Work out the finished part from the listing and answer in its coordinate system (mm). Face numbers are marked on the shaded views. A direction names the side the tool comes from. Coordinates: 2 decimals unless noted, no trailing zeros. Write each loop counter-clockwise with the first axis right and the second up, starting at its lowest first coordinate (ties: lowest second). Pieces come first, ordered by that corner, then holes. Notation, with made-up numbers: (-23, 6.25) - (29, 6.25) arc R20 ccw to (29, 22.25) - close; hole circle Ø9 at (21.5, -31.5). An arc over 180 degrees is marked (long way). One line per item, written item: value.
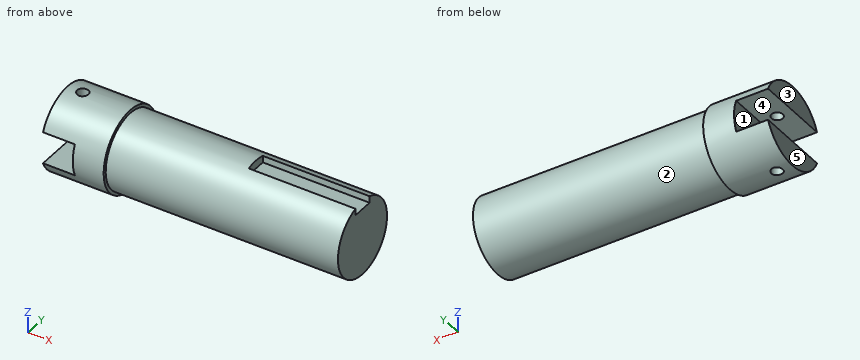
```python
from build123d import *

# Parameters (mm, degrees)
SKETCH1_R               = 30
BOSS_EXTRUDE1_DEPTH     = 185
SKETCH2_R               = 32.5
BOSS_EXTRUDE2_DEPTH     = 50
SKETCH3_W               = 17.227034698
SKETCH3_H               = 11
CUT_EXTRUDE1_DEPTH      = 85
SKETCH6_W               = 97.129715822
SKETCH6_H               = 25.4
CUT_EXTRUDE2_DEPTH      = 25.4
CUT_EXTRUDE3_DEPTH      = 66.4
CUT_EXTRUDE3_DEPTH_BACK = 25.4
SKETCH7_R               = 4.5


with BuildPart() as part:
    # Sketch1 → Boss-Extrude1 (new body)
    with BuildSketch(Plane.YZ):
        with Locations(Location((0, 0, 0), (0, 0, 270))):
            Circle(SKETCH1_R)
    extrude(amount=BOSS_EXTRUDE1_DEPTH)

    # Sketch2 → Boss-Extrude2 (add)
    with BuildSketch(Plane.ZY):
        Circle(SKETCH2_R)
    extrude(amount=BOSS_EXTRUDE2_DEPTH)

    # Sketch3 → Cut-Extrude1 (cut)
    with BuildSketch(Plane.YZ.offset(185)):
        with Locations((0, 28.9)):
            Rectangle(SKETCH3_W, SKETCH3_H)
    extrude(amount=-CUT_EXTRUDE1_DEPTH, mode=Mode.SUBTRACT)

    # Sketch6 → Cut-Extrude2 (cut)
    with BuildSketch(Plane(origin=(-50, 0, 0), x_dir=(0, -1, 0), z_dir=(-1, 0, 0))):
        with Locations((3.400411954, 0)):
            Rectangle(SKETCH6_W, SKETCH6_H)
    extrude(amount=-CUT_EXTRUDE2_DEPTH, mode=Mode.SUBTRACT)

    # Sketch7 → Cut-Extrude3 (cut, two sides: drawn at the far end of the back side and taken through both)
    with BuildSketch(Plane.XY.offset(-12.7).offset(-CUT_EXTRUDE3_DEPTH_BACK)):
        with Locations(Location((-37.729755698, 0, 0), (0, 0, 180))):
            Circle(SKETCH7_R)
    extrude(amount=CUT_EXTRUDE3_DEPTH + CUT_EXTRUDE3_DEPTH_BACK, mode=Mode.SUBTRACT)


solid = part.part
```
Item 1: Given pin 1 (10 mm diameter, centred on x = -0.5, y = 20, fed in from +Z); pin 2 (4.5 mm diameter, centred on x = 149.5, z = 26.5, fed in from -Y); pin 3 (3 mm diameter, centred on y = -18.5, z = 2, fed in from -X); pin 4 (7 mm diameter, centred on x = -37.73, y = 0, fed in from +Z), each flat-ended and moving along its own axis, determine where each tip first touches the part or whether it passes through.
Evaluation:
pin 1: stops at z = 28.83
pin 2: stops at y = -17.66
pin 3: stops at x = -24.6
pin 4: passes through
Item 2: Section D-D, the plane x = 53 is taken. Determine the outline of the cut face in (y, z).
Evaluation:
outline: circle Ø60 at (0, 0)
Item 3: Section A-A, the plane y = 0 is taken. Determine the outline of the cut face in (x, z).
Evaluation:
outline: (-50, -32.5) - (-42.23, -32.5) - (-42.23, -12.7) - (-50, -12.7) - close; (-50, 12.7) - (-42.23, 12.7) - (-42.23, 32.5) - (-50, 32.5) - close; (-33.23, -32.5) - (0, -32.5) - (0, -30) - (185, -30) - (185, 23.4) - (100, 23.4) - (100, 30) - (0, 30) - (0, 32.5) - (-33.23, 32.5) - (-33.23, 12.7) - (-24.6, 12.7) - (-24.6, -12.7) - (-33.23, -12.7) - close
Item 4: Which of the six approach directions +Z, -Z, +X, -X, +Y, -Y give full straight-line access (tool end or side, diameter ignored) to the marked faces 4 and 5?
Evaluation:
face 4: -X, +Y, -Y
face 5: +Z, -Z, -X, +Y, -Y
Item 5: Consider probe 1 along X at (y, z) = (29, 12); probe 2 along Y at (x, z) = (170, 2); probe 3 along X at (y, z) = (-22.5, 23). Determine where each line is inside the solid, lowest interval first.
Evaluation:
probe 1: x = -24.6 to 0
probe 2: y = -29.93 to 29.93
probe 3: x = -50 to 0
Item 6: Section C-C, the plane z = 0 is taken. Determine the outline of the cut face in (x, y), then the cut area to 3 significant figures.
Evaluation:
outline: (-24.6, -32.5) - (0, -32.5) - (0, -30) - (185, -30) - (185, 30) - (0, 30) - (0, 32.5) - (-24.6, 32.5) - close
area: 12,700 mm2
Item 7: Determine the mould class of the marked faces 1, 2 and 3 for opening direction Z: +Z half, -Z half, draft (parallel to the pull), parting line (faces both ways), or undercut.
Evaluation:
face 1: undercut
face 2: parting line
face 3: draft
Item 8: Section B-B, the plane z = -26 is taken. Determine the outline of the cut face in (x, y), then the cut area to 3 significant figures.
Evaluation:
outline: (-50, -19.5) - (0, -19.5) - (0, -14.97) - (185, -14.97) - (185, 14.97) - (0, 14.97) - (0, 19.5) - (-50, 19.5) - close; hole circle Ø9 at (-37.73, 0)
area: 7,420 mm2
